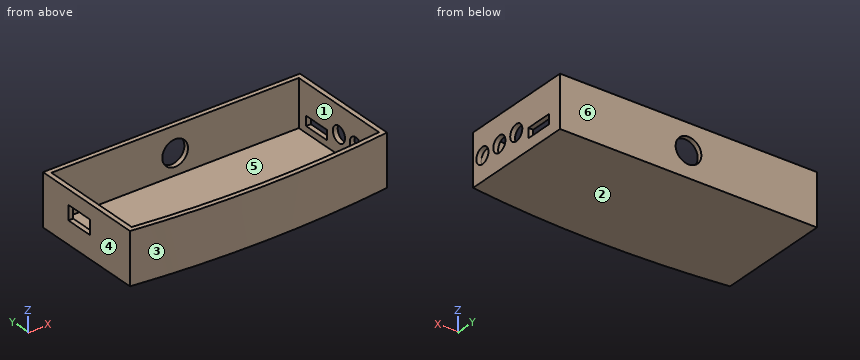
```python
from build123d import *

# Parameters (mm, degrees)
SKETCH_1_W          = 80
SKETCH_1_H          = 36
EXTRUDE_1_DEPTH     = 16
SHELL_1_T           = -1.5
CUT_EXTRUDE_3_REACH = 89.695
SKETCH_2_W          = 4.5
SKETCH_2_H          = 9
CUT_EXTRUDE_4_REACH = 89.695
SKETCH_6_R          = 2.5
SKETCH_6_W          = 3
SKETCH_6_H          = 8.6
SKETCH_7_R          = 4
CUT_EXTRUDE_5_DEPTH = 2


with BuildPart() as part:
    # 草图1 → 凸台-拉伸1 (new body)
    with BuildSketch(Plane.XY):
        with Locations((-50.420566467, -11.667328482)):
            Rectangle(SKETCH_1_W, SKETCH_1_H)
        with BuildLine():
            Line((-10.420566467, -29.667328482), (-90.420566467, -29.667328482))
            ThreePointArc((-90.420566467, -29.667328482), (-50.420566467, -32.163413079), (-10.420566467, -29.667328482))
        make_face()
    extrude(amount=EXTRUDE_1_DEPTH)

    # 抽壳1
    shell_1_openings = [part.faces().sort_by_distance(p)[0] for p in [
        (-50.420566467, -12.507347913, 16),
    ]]
    offset(amount=SHELL_1_T, openings=shell_1_openings, kind=Kind.INTERSECTION)

    # 草图2 → 切除-拉伸3 (cut, up to next)
    with BuildSketch(Plane.ZY.offset(90.420566467), mode=Mode.PRIVATE) as cut_extrude_3_sk1:
        with Locations((9.25, -8.667328482)):
            Rectangle(SKETCH_2_W, SKETCH_2_H)
    cut_extrude_3_tool1 = extrude(cut_extrude_3_sk1.sketch, amount=-CUT_EXTRUDE_3_REACH, mode=Mode.PRIVATE) & part.part
    add(cut_extrude_3_tool1.solids().sort_by_distance((-90.420566, -8.667328, 9.25))[0], mode=Mode.SUBTRACT)

    # 草图6 → 切除-拉伸4 (cut, up to next)
    with BuildSketch(Plane(origin=(-10.420566467, 0, 0), x_dir=(0, 0, -1), z_dir=(1, 0, 0)), mode=Mode.PRIVATE) as cut_extrude_4_sk1:
        with Locations((-7.5, -11.767328482)):
            Circle(SKETCH_6_R)
    cut_extrude_4_tool1 = extrude(cut_extrude_4_sk1.sketch, amount=-CUT_EXTRUDE_4_REACH, mode=Mode.PRIVATE) & part.part
    # 草图6 → 切除-拉伸4 (cut, up to next)
    with BuildSketch(Plane(origin=(-10.420566467, 0, 0), x_dir=(0, 0, -1), z_dir=(1, 0, 0)), mode=Mode.PRIVATE) as cut_extrude_4_sk2:
        with Locations((-7.5, -18.767328482)):
            Circle(SKETCH_6_R)
    cut_extrude_4_tool2 = extrude(cut_extrude_4_sk2.sketch, amount=-CUT_EXTRUDE_4_REACH, mode=Mode.PRIVATE) & part.part
    # 草图6 → 切除-拉伸4 (cut, up to next)
    with BuildSketch(Plane(origin=(-10.420566467, 0, 0), x_dir=(0, 0, -1), z_dir=(1, 0, 0)), mode=Mode.PRIVATE) as cut_extrude_4_sk3:
        with Locations((-7.5, -25.767328482)):
            Circle(SKETCH_6_R)
    cut_extrude_4_tool3 = extrude(cut_extrude_4_sk3.sketch, amount=-CUT_EXTRUDE_4_REACH, mode=Mode.PRIVATE) & part.part
    # 草图6 → 切除-拉伸4 (cut, up to next)
    with BuildSketch(Plane(origin=(-10.420566467, 0, 0), x_dir=(0, 0, -1), z_dir=(1, 0, 0)), mode=Mode.PRIVATE) as cut_extrude_4_sk4:
        with Locations((-5, -2.467328482)):
            Rectangle(SKETCH_6_W, SKETCH_6_H)
    cut_extrude_4_tool4 = extrude(cut_extrude_4_sk4.sketch, amount=-CUT_EXTRUDE_4_REACH, mode=Mode.PRIVATE) & part.part
    add(cut_extrude_4_tool1.solids().sort_by_distance((-10.420566, -11.767328, 7.5))[0], mode=Mode.SUBTRACT)
    add(cut_extrude_4_tool2.solids().sort_by_distance((-10.420566, -18.767328, 7.5))[0], mode=Mode.SUBTRACT)
    add(cut_extrude_4_tool3.solids().sort_by_distance((-10.420566, -25.767328, 7.5))[0], mode=Mode.SUBTRACT)
    add(cut_extrude_4_tool4.solids().sort_by_distance((-10.420566, -2.467328, 5))[0], mode=Mode.SUBTRACT)

    # 草图7 → 切除-拉伸5 (cut)
    with BuildSketch(Plane(origin=(0, 6.332671518, 0), x_dir=(1, 0, 0), z_dir=(0, 1, 0))):
        with Locations(Location((-50.420566467, -8, 0), (0, 0, 270))):
            Circle(SKETCH_7_R)
    extrude(amount=-CUT_EXTRUDE_5_DEPTH, mode=Mode.SUBTRACT)


solid = part.part
```
Design review of the part built by this model. Coordinates are the model's own, in mm. Face numbers are marked on the shaded views. A direction names the side the tool comes from. Give positions to 0.01 mm unless a question says otherwise; leave off trailing zeros. Write each loop counter-clockwise with the first axis right and the second up, starting at its lowest first coordinate (ties: lowest second). Pieces come first, ordered by that corner, then holes. Notation, with made-up numbers: (4.25, -30.75) - (45.25, -30.75) arc R17 cw to (45.25, 2.25) - close; hole circle Ø2 at (2, 1.5). An arc over 180 degrees is marked (long way). Return JSON: item names as keys, results as strings. Group by question number.
(1) We need section A-A, the plane z = 13.75. Give the boundary of the cut face in (x, y).
(2) To check wall thickness, follow probe 1 along X at (y, z) = (2.5, 15); probe 2 along Y at (x, z) = (-50.5, 13.5); probe 3 along Z at (x, y) = (-58, -26.5). State the ranges of each line that lie inside material, in increasing order.
(3) We need section C-C, the plane z = 9. Give the boundary of the cut face in (x, y), then the cut area to 3 significant figures.
(4) Machinability: for the marked faces 1 and 2, which of the approach directions +Z, -Z, +X, -X, +Y, -Y give a long, thin tool a straight path to every point of the face, cutting with its end or side? Answer none if there is none.
(5) We need section B-B, the plane x = -47.5. Give the boundary of the cut face in (y, z), then the cut area to 3 significant figures.
(6) Mouldability with a two-part tool opening along X and no side actions: class the marked faces 3, 4, 5 and 6 as +X half, -X half, draft (parallel to the pull), parting line (faces both ways), or undercut.
(7) Insertion check: pin 1 (1.5 mm diameter, centred on x = -77, y = -14, fed in from -Z); pin 2 (6.5 mm diameter, centred on x = -50.42, z = 8, fed in from +Y); pin 3 (5 mm diameter, centred on x = -59, y = 1, fed in from +Z); pin 4 (4 mm diameter, centred on y = -11.77, z = 7.5, fed in from +X). Each pin has a flat end and moves straight along its axis. Give the tip position at first contact, or say it passes through.
(8) We need section D-D, the plane y = -24. Give the boundary of the cut face in (x, z).
Reported:
{
 "1": {"outline": "(-90.42, -29.67) arc R321.75 ccw to (-10.42, -29.67) - (-10.42, 6.33) - (-90.42, 6.33) - close; hole (-88.92, -28.34) arc R320.25 ccw to (-11.92, -28.34) - (-11.92, 4.83) - (-88.92, 4.83) - close"},
 "2": {"probe 1": "x = -90.42 to -88.92, -11.92 to -10.42", "probe 2": "y = -32.16 to -30.66, 4.83 to 6.33", "probe 3": "z = 0 to 1.5"},
 "3": {"outline": "(-90.42, -29.67) arc R321.75 ccw to (-10.42, -29.67) - (-10.42, -27.77) - (-11.92, -27.77) - (-11.92, -28.34) arc R320.25 cw to (-88.92, -28.34) - (-88.92, -13.17) - (-90.42, -13.17) - close; (-90.42, -4.17) - (-88.92, -4.17) - (-88.92, 4.83) - (-54.29, 4.83) - (-54.29, 6.33) - (-90.42, 6.33) - close; (-46.55, 4.83) - (-11.92, 4.83) - (-11.92, -9.77) - (-10.42, -9.77) - (-10.42, 6.33) - (-46.55, 6.33) - close; (-11.92, -23.77) - (-10.42, -23.77) - (-10.42, -20.77) - (-11.92, -20.77) - close; (-11.92, -16.77) - (-10.42, -16.77) - (-10.42, -13.77) - (-11.92, -13.77) - close", "area": "296 mm2"},
 "4": {"face 1": "+Z", "face 2": "-Z, +X, -X, +Y, -Y"},
 "5": {"outline": "(-32.15, 0) - (6.33, 0) - (6.33, 5.27) - (4.83, 5.27) - (4.83, 1.5) - (-30.65, 1.5) - (-30.65, 16) - (-32.15, 16) - close; (4.83, 10.73) - (6.33, 10.73) - (6.33, 16) - (4.83, 16) - close", "area": "93.0 mm2"},
 "6": {"face 3": "parting line", "face 4": "-X half", "face 5": "undercut", "face 6": "draft"},
 "7": {"pin 1": "stops at z = 0", "pin 2": "stops at y = -30.65", "pin 3": "stops at z = 1.5", "pin 4": "stops at x = -88.92"},
 "8": {"outline": "(-90.42, 0) - (-10.42, 0) - (-10.42, 5.73) - (-11.92, 5.73) - (-11.92, 1.5) - (-88.92, 1.5) - (-88.92, 16) - (-90.42, 16) - close; (-11.92, 9.27) - (-10.42, 9.27) - (-10.42, 16) - (-11.92, 16) - close"}
}
